Here's how the part is built. I have some questions about the finished solid (model axes, mm). Face numbers are marked on the shaded views. A direction names the side the tool comes from. Round coordinates to 2 decimals unless told otherwise and drop trailing zeros. Write each loop counter-clockwise with the first axis right and the second up, starting at its lowest first coordinate (ties: lowest second). Pieces come first, ordered by that corner, then holes. Notation, with made-up numbers: (31, 49) - (85, 49) arc R24 cw to (85, 87) - close; hole circle Ø4 at (41.5, 39.5). An arc over 180 degrees is marked (long way). Use one line per item in the form item = value. Start each with the question number.
1. If I drill on line 1 along Z through (x, y) = (36, 116.5); line 2 along Z through (x, y) = (40.5, 170.5); line 3 along Z through (x, y) = (60.5, 136), over which ranges is the centre line in solid material (lowest first)?
2. I want a section at C-C, the plane x = 9. State how many separate pieces and enclosed holes the cut face has, plus the area to 3 significant figures.
3. Which directions (+Z, -Z, +X, -X, +Y, -Y) give clear straight access to the entire face, cutting with the end or side of a thin tool? Please do the marked faces 1, 2, 3, 4 and 5.
4. We'd pull the mould along X, two halves only. Please class the marked faces 6, 7 and 8: +X half, -X half, draft (parallel to the pull), parting line (faces both ways), or undercut.
5. Will these pins go through, and if not, where does the flat tip stop? pin 1 (8.5 mm diameter, centred on x = 53.5, y = 194, fed in from +Z); pin 2 (1.5 mm diameter, centred on x = 8, y = 107.5, fed in from -Z); pin 3 (1.1 mm diameter, centred on y = 149, z = 43, fed in from +X).
6. I want a section at A-A, the plane x = 68. List the corners of the cut face in (y, z) for me.
7. I want a section at B-B, the plane z = 9.5. List the corners of the cut face in (x, y) for me, plus the area to 3 significant figures.
```python
from build123d import *

# Parameters (mm, degrees)
PAD066_DEPTH        = 140.15
POCKET025_DEPTH     = 42.751
POCKET026_DEPTH     = 4.25
LINEARPATTERN_COUNT = 10
LINEARPATTERN_PITCH = 5.8055555556


with BuildPart() as part:
    # Sketch109 (on DatumPlane) → Pad066 (new body)
    with BuildSketch(Plane.XZ.offset(-232.15)):
        Polygon((-1.5, 44.35), (44, 44.35), (45, 43.35), (45, 42.35), (61.7, 42.35), (58.9121410033, 41.05), (53.9996494638, 41.05), (51.7, 40.05), (53.9996494638, 39.65), (56.2992989276, 39.25), (60.2, 39.25), (61.7, 37.75), (51.907721902, 37.75), (49.6346030244, 38.2803944048), (47.2, 36.794745537), (61.0928843686, 33.5530725177), (62.7, 31.6377866903), (49.6346030244, 34.6863793179), (47.2, 33.2007304502), (61.0928843686, 29.9590574308), (62.7, 28.0437716034), (49.6346030244, 31.0923642311), (47.2, 29.35), (74.5, 22.98), (74.5, 13.6), (62, 13.6), (62, 1.6), (48, 1.6), (48, 14.6), (32.5, 14.6), (32.5, 16.6), (34, 16.6), (32.5, 18.1), (34, 18.1), (35.5, 16.6), (38.5, 16.6), (37, 18.1), (38.5, 18.1), (40, 16.6), (43, 16.6), (41.5, 18.1), (43, 18.1), (44.5, 16.6), (47.5, 16.6), (46, 18.1), (47.5, 18.1), (49, 16.6), (52, 16.6), (50.5, 18.1), (52, 18.1), (53.5, 16.6), (56.5, 16.6), (55, 18.1), (56.5, 18.1), (58, 16.6), (69.5, 16.6), (69.5, 20.6), (48.5, 25.5), (33.5, 25.5), (33.5, 30.6), (37.5, 30.6), (42, 32.35), (33.5, 32.35), (31.5, 34), (37.5, 34), (42, 35.75), (31.5, 35.75), (31.5, 39.35), (12.5, 39.35), (12.5, 42.35), (-1.5, 42.35), align=None)
    extrude(amount=PAD066_DEPTH)

    # Sketch110 (on Face2 of Pad066) → Pocket025 (cut, through all)
    with BuildSketch(Plane(origin=(0, 232.15, 44.35), x_dir=(1, 0, 0), z_dir=(0, 0, 1))):
        Polygon((46, -161.7962), (46, -119.15), (63.5398448916, -119.15), (102.309495165, -80.3803497266), (102.309495165, -161.7962), align=None)
        Polygon((15.2813043199, 6.9694708626), (137.7083776888, -49.0965638734), (137.7083776888, 6.9694708626), align=None)
    extrude(amount=-POCKET025_DEPTH, mode=Mode.SUBTRACT)

    # Sketch111 (on Face2 of Pocket025) → Pocket026 (cut)
    with BuildSketch(Plane(origin=(0, 232.15, 44.35), x_dir=(1, 0, 0), z_dir=(0, 0, 1))):
        Polygon((-49.9825431556, -63.9110456519), (101.4245877181, -154.7553241761), (95.6823064576, -152.7093838745), (-60.3201060514, -59.1079363692), align=None)
    pocket026 = extrude(amount=-POCKET026_DEPTH, mode=Mode.SUBTRACT)

    # LinearPattern: Pocket026 ×10
    with Locations(*[(0, i * LINEARPATTERN_PITCH, 0) for i in range(1, LINEARPATTERN_COUNT)]):
        add(pocket026, mode=Mode.SUBTRACT)


solid = part.part
```
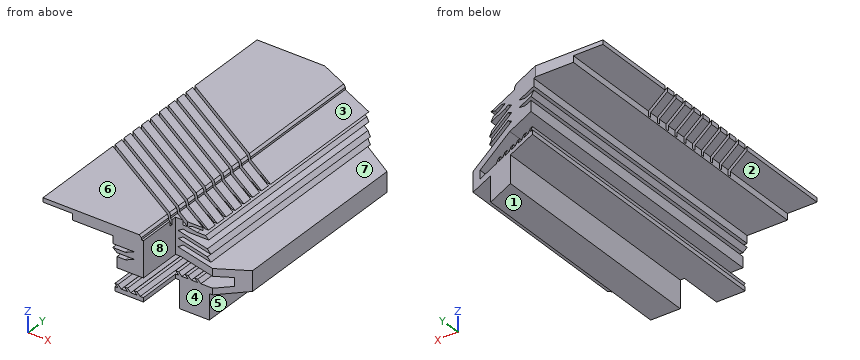
Model answer:
q1.line_1 = 14.6 to 16.6, 25.5 to 30.6, 32.35 to 34, 35.75 to 40.1
q1.line_2 = 14.6 to 16.6, 25.5 to 31.77, 32.35 to 35.17, 35.75 to 44.35
q1.line_3 = 1.6 to 16.6, 22.7 to 26.25, 28.56 to 30.1, 32.15 to 33.69, 37.75 to 38.95
q2.separate_pieces = 11
q2.enclosed_holes = 0
q2.area = 252 mm2
q3.face_1 = -Z, +X, -X, +Y, -Y
q3.face_2 = -Z, -X, +Y, -Y
q3.face_3 = +Z, +X, +Y, -Y
q3.face_4 = +Z, -Z, +X, -Y
q3.face_5 = -Z, +X, +Y, -Y
q4.face_6 = draft
q4.face_7 = undercut
q4.face_8 = +X half
q5.pin_1 = 42.35
q5.pin_2 = 42.35
q5.pin_3 = 45
q6.outline = (117.46, 13.6) - (214.98, 13.6) - (214.98, 16.6) - (117.46, 16.6) - close; (117.46, 20.95) - (214.98, 20.95) - (214.98, 24.5) - (117.46, 24.5) - close
q7.outline = (48, 113) - (62, 113) - (62, 217.72) - (48, 224.14) - close
q7.area = 1,510 mm2
